Model file for the job. Use its own axes, mm. Face numbers are marked on the shaded views. A direction names the side the tool comes from. Round coordinates to 2 decimals unless told otherwise and drop trailing zeros. Loops run counter-clockwise (first coordinate to the right, second up) from the corner with the lowest first, then second, coordinate; pieces in that order, holes last. Notation, with made-up numbers: (31.5, 86) - (49.5, 86) arc R19 cw to (49.5, 117) - close; hole circle Ø2 at (13, 78). An arc over 180 degrees is marked (long way). Answer as a JSON object with one key per item and string values.
from build123d import *

# Parameters (mm, degrees)
SKETCH1_W                 = 17.5
SKETCH1_H                 = 55
BASE_FLANGE1_DEPTH        = 2
SKETCHED_START            = -23.286713287
SKETCHED_BEND3_DEPTH      = 17.5
SKETCHED_BEND3_2_DEPTH    = 17.5
F_4_CLEARANCE_HOLE1_D     = 3.2639
F_4_CLEARANCE_HOLE1_DEPTH = 2
F_4_CLEARANCE_HOLE1_TIP   = 0.980574487


# Read off the part's stored shape, not the designer's step: Sketched Bend3
# Sheet-metal steps are written as plain solids
with BuildPart() as part:
    # Sketch1 → Base-Flange1 (new body)
    with BuildSketch(Plane(origin=(0, 0, 0), x_dir=(1, 0, 0), z_dir=(0, 1, 0))):
        with Locations((-14.536713287, -6.17016317)):
            Rectangle(SKETCH1_W, SKETCH1_H)
    extrude(amount=-BASE_FLANGE1_DEPTH)

    # Sketched Bend3 outline → Sketched Bend3 (cut)
    with BuildSketch(Plane.YZ.offset(SKETCHED_START)):
        with BuildLine():
            ThreePointArc((-2, -11.32983683), (-1.443395312, -9.675569621), (0, -8.694234432))
            Line((0, -8.694234432), (0, 33.67016317))
            Line((0, 33.67016317), (-2, 33.67016317))
            Line((-2, 33.67016317), (-2, -11.32983683))
        make_face()
    extrude(amount=SKETCHED_BEND3_DEPTH, mode=Mode.SUBTRACT)

    # Sketched Bend3 2 outline → Sketched Bend3 2 (add)
    with BuildSketch(Plane.YZ.offset(SKETCHED_START)):
        with BuildLine():
            ThreePointArc((0, -11.32983683), (0.215745145, -10.808981975), (0.7366, -10.59323683))
            Line((0.7366, -10.59323683), (43.197250658, -10.59323683))
            Line((43.197250658, -10.59323683), (43.197250658, -8.59323683))
            Line((43.197250658, -8.59323683), (0.7366, -8.59323683))
            ThreePointArc((0.7366, -8.59323683), (0.364854094, -8.6186038), (0, -8.694234432))
            Line((0, -8.694234432), (0, -11.32983683))
        make_face()
    extrude(amount=SKETCHED_BEND3_2_DEPTH)

    # #4 Clearance Hole1
    with Locations(Plane.XZ.offset(2)):
        with Locations((-9.786713287, -16.32983683), (-19.286713287, -16.32983683)):
            Hole(F_4_CLEARANCE_HOLE1_D / 2, depth=F_4_CLEARANCE_HOLE1_DEPTH)
            with Locations((0, 0, -(F_4_CLEARANCE_HOLE1_DEPTH + F_4_CLEARANCE_HOLE1_TIP / 2))):  # 118° drill point
                Cone(0, F_4_CLEARANCE_HOLE1_D / 2, F_4_CLEARANCE_HOLE1_TIP, mode=Mode.SUBTRACT)


solid = part.part
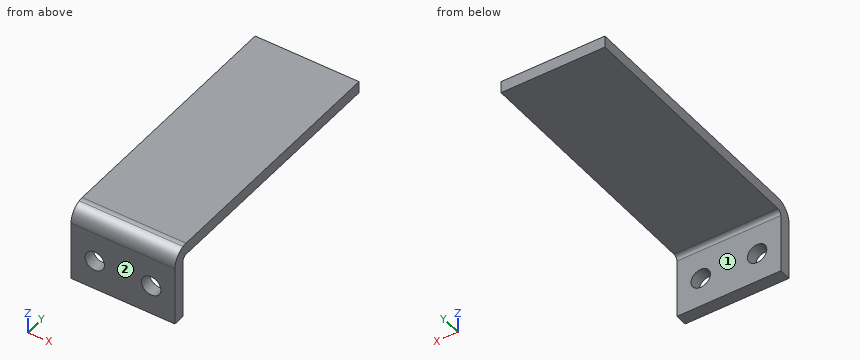
1) Slice it at A-A on x = -14.25. List the corners of the cut face in (y, z), then the cut area to 3 significant figures.
Values follow:
{"outline": "(-2, -21.33) - (0, -21.33) - (0, -11.33) arc R0.74 cw to (0.74, -10.59) - (43.2, -10.59) - (43.2, -8.59) - (0.74, -8.59) arc R2.74 ccw to (-2, -11.33) - close", "area": "110 mm²"}
2) Slice it at C-C on y = 37. List the corners of the cut face in (x, z).
Values follow:
{"outline": "(-23.29, -10.59) - (-5.79, -10.59) - (-5.79, -8.59) - (-23.29, -8.59) - close"}
3) Probe probe 1 along Y at (x, z) = (-7.25, -17.25); probe 2 along Z at (x, y) = (-18.5, 2.5); probe 3 along Y at (x, z) = (-19.5, -10.5). List the from-to ranges inside material, lowest first.
Values follow:
{"probe 1": "-2 to 0", "probe 2": "-10.59 to -8.59", "probe 3": "-1.87 to 43.2"}
4) Drop flat-ended pins along their axis: P1, Ø4, axis at y = 29, z = -14, coming from the -X side; P2, Ø4, axis at x = -19.29, z = -16.33, coming from the +Y side; P3, Ø4, axis at x = -9.79, z = -16.33, coming from the -Y side. Give the stop position or say it passes through.
Values follow:
{"P1": "through", "P2": "y = 0", "P3": "y = -2"}
5) Tool access for the marked faces 1 and 2: list every direction of +Z, -Z, +X, -X, +Y, -Y with a clear straight run to the whole face (end or side of a thin tool).
Values follow:
{"face 1": "-Z, +X, -X, +Y", "face 2": "+Z, -Z, +X, -X, -Y"}
6) Slice it at B-B on z = -12.75. List the corners of the cut face in (x, y).
Values follow:
{"outline": "(-23.29, -2) - (-5.79, -2) - (-5.79, 0) - (-23.29, 0) - close"}
